Design review of the part shown in the three views and the two pictorial views. Dimensions are in mm from the part's minimum x, y and z. Round coordinates to 2 decimals unless told otherwise and drop trailing zeros. Order: outer loops, then holes, each group sorted by start corner. A loop starts at its lowest first (then second) coordinate and runs counter-clockwise, first axis right, second up. Notation, with made-up numbers: (61.25, 87.5) -> (97.25, 87.5) arc R18 ccw to (97.25, 97.5) -> close; hole circle Ø5 at (82, 7.25). An arc over 180 degrees is marked (long way). Put each result on its own line as item: value. Start each with the question number.
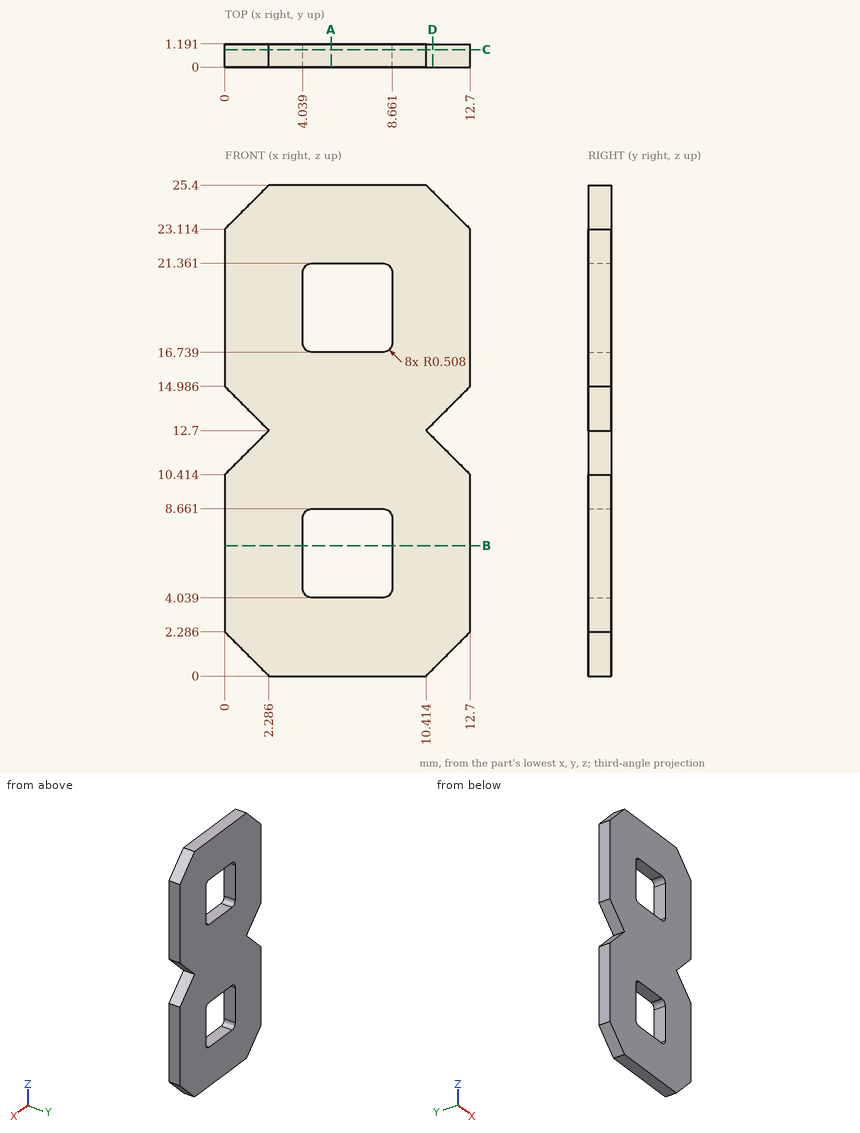
Q1. Take a section at A-A on x = 5.5. Give the boundary of the cut face in (y, z).
Q2. Wall thickness on probe 1 along Z at (x, y) = (5.5, 0.95); probe 2 along X at (y, z) = (0.95, 18.75); probe 3 along Z at (x, y) = (2, 1) (1 decimal): over which ranges is each line inside the solid? List them lowest first. Write a range as [from, to].
Q3. Take a section at B-B on z = 6.75. Give the boundary of the cut face in (x, y).
Q4. Take a section at D-D on x = 10.75. Give the boundary of the cut face in (y, z).
Q5. Take a section at C-C on y = 0.9. State how many separate pieces and enclosed holes the cut face has, and give its area (3 significant figures).
Calculated:
1. outline: (0, 0) -> (1.19, 0) -> (1.19, 4.04) -> (0, 4.04) -> close; (0, 8.66) -> (1.19, 8.66) -> (1.19, 16.74) -> (0, 16.74) -> close; (0, 21.36) -> (1.19, 21.36) -> (1.19, 25.4) -> (0, 25.4) -> close
2. probe 1: z = [0, 4.04], [8.66, 16.74], [21.36, 25.4]
2. probe 2: x = [0, 4.04], [8.66, 12.7]
2. probe 3: z = [0.3, 12.4], [13, 25.1]
3. outline: (0, 0) -> (4.04, 0) -> (4.04, 1.19) -> (0, 1.19) -> close; (8.66, 0) -> (12.7, 0) -> (12.7, 1.19) -> (8.66, 1.19) -> close
4. outline: (0, 0.34) -> (1.19, 0.34) -> (1.19, 12.36) -> (0, 12.36) -> close; (0, 13.04) -> (1.19, 13.04) -> (1.19, 25.06) -> (0, 25.06) -> close
5. separate pieces: 1
5. enclosed holes: 2
5. area: 259 mm²
